Part model, mm, in its own coordinate system. Coordinates: 2 decimals unless noted, no trailing zeros. Loops run counter-clockwise (first coordinate to the right, second up) from the corner with the lowest first, then second, coordinate; pieces in that order, holes last. Notation, with made-up numbers: (-7, 82.5) - (22, 82.5) arc R11 ccw to (22, 101.5) - close; hole circle Ø11 at (80.5, 69). An arc over 180 degrees is marked (long way). Use a Markdown table: item, result. Add a question column.
1) Drop a flat-ended pin along its axis: P1, Ø6, axis at x = 29.19, y = -29.19, coming from the +Z side. Give the stop position or say it passes through.
2) Pull direction X, two halves, no side cores. Call faces 1 (the face through (-38.711, 0, 2)), 2 (the face through (33.6, -33.75, 1.57)), 3 (the face through (29.71, -31.54, 0.34)): +X half, -X half, draft (parallel to the pull), parting line (faces both ways), or undercut.
3) Probe probe 1 along Y at (x, z) = (-28, 0.5); probe 2 along X at (y, z) = (29, 0.35); probe 3 along Y at (x, z) = (-32, 3). List the from-to ranges inside material, lowest first. Write a range as [from, to].
4) Band-saw the part on A-A (z = 0.85). Give the cut face in (x, y) (3 decimals).
from build123d import *

# Parameters (mm, degrees)
SKETCH1_R           = 47.625
BOSS_EXTRUDE1_DEPTH = 3.175
CIRPATTERN1_COUNT   = 4
SKETCH6_OUTSIDE_W   = 124.198
SKETCH6_OUTSIDE_H   = 124.198
SKETCH6_OUTSIDE_W_2 = 77.421664786
SKETCH6_OUTSIDE_H_2 = 77.421664786
CUT_EXTRUDE2_DEPTH  = 68.426714847


with BuildPart() as part:
    # Sketch1 → Boss-Extrude1 (new body)
    with BuildSketch(Plane.XY):
        Circle(SKETCH1_R)
    extrude(amount=BOSS_EXTRUDE1_DEPTH)

    # Sketch3 → CSK for #8 Flat Head Machine Screw1 (revolve, cut)
    with BuildSketch(Plane(origin=(29.185832393, 29.185832393, 3.175), x_dir=(0, -1, 0), z_dir=(1, 0, 0))):
        Polygon((0, 0), (0, 3.175), (2.2479, 3.175), (2.2479, 3.026511835), (4.8788066, 0), align=None)
    csk_for_8_flat_head_machine_screw1 = revolve(axis=Axis((29.185832393, 29.185832393, 9.525), (0, 0, -1)), mode=Mode.SUBTRACT)

    # CirPattern1: CSK for #8 Flat Head Machine Screw1 ×4 about axis
    cirpattern1_axis = Axis((0, 0, 0), (0, 0, 1))
    for i in range(1, CIRPATTERN1_COUNT):
        add(csk_for_8_flat_head_machine_screw1.rotate(cirpattern1_axis, i * 360 / CIRPATTERN1_COUNT), mode=Mode.SUBTRACT)

    # Sketch6 outside → Cut-Extrude2 (cut, through all)
    with BuildSketch(Plane.XY.offset(3.175)):
        Rectangle(SKETCH6_OUTSIDE_W, SKETCH6_OUTSIDE_H)
        Rectangle(SKETCH6_OUTSIDE_W_2, SKETCH6_OUTSIDE_H_2, mode=Mode.SUBTRACT)
    extrude(amount=-CUT_EXTRUDE2_DEPTH, mode=Mode.SUBTRACT)


solid = part.part
Answer block:
| question | item | result |
|---|---|---|
| 1 | P1 | z = 1.02 |
| 2 | face 1 | -X half |
| 2 | face 2 | +X half |
| 2 | face 3 | undercut |
| 3 | probe 1 | [-38.52, -31.45], [-26.92, 26.92], [31.45, 38.52] |
| 3 | probe 2 | [-37.78, -31.6], [-26.77, 26.77], [31.6, 37.78] |
| 3 | probe 3 | [-35.27, -32.98], [-25.39, 25.39], [32.98, 35.27] |
| 4 | outline | (-38.711, -27.742) arc R47.625 ccw to (-27.742, -38.711) - (27.742, -38.711) arc R47.625 ccw to (38.711, -27.742) - (38.711, 27.742) arc R47.625 ccw to (27.742, 38.711) - (-27.742, 38.711) arc R47.625 ccw to (-38.711, 27.742) - close; hole circle Ø5.715 at (-29.186, -29.186); hole circle Ø5.715 at (-29.186, 29.186); hole circle Ø5.715 at (29.186, -29.186); hole circle Ø5.715 at (29.186, 29.186) |
